Build history of the part. All positions in model axes, mm. Face numbers are marked on the shaded views. Give positions to 0.01 mm unless a question says otherwise; leave off trailing zeros. Write each loop counter-clockwise with the first axis right and the second up, starting at its lowest first coordinate (ties: lowest second). Pieces come first, ordered by that corner, then holes.
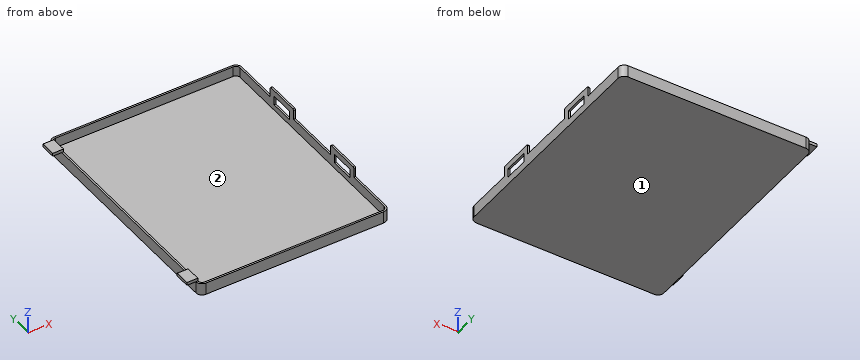
from build123d import *

# Parameters (mm, degrees)
BOSS_EXTRUDE1_DEPTH = 2
SHELL1_T            = -0.3
BOSS_EXTRUDE2_DEPTH = 0.3
SKETCH3_W           = 0.75
SKETCH3_H           = 4
CUT_EXTRUDE1_DEPTH  = 0.3
FILLET1_R           = 0.2
BOSS_EXTRUDE4_DEPTH = 0.5


with BuildPart() as part:
    # Sketch1 → Boss-Extrude1 (new body)
    with BuildSketch(Plane.XY):
        with BuildLine():
            Line((-14.75, 19.5), (14.75, 19.5))
            ThreePointArc((14.75, 19.5), (15.457106781, 19.207106781), (15.75, 18.5))
            Line((15.75, 18.5), (15.75, -18.5))
            ThreePointArc((15.75, -18.5), (15.457106781, -19.207106781), (14.75, -19.5))
            Line((14.75, -19.5), (-14.75, -19.5))
            ThreePointArc((-14.75, -19.5), (-15.457106781, -19.207106781), (-15.75, -18.5))
            Line((-15.75, -18.5), (-15.75, 18.5))
            ThreePointArc((-15.75, 18.5), (-15.457106781, 19.207106781), (-14.75, 19.5))
        make_face()
    extrude(amount=BOSS_EXTRUDE1_DEPTH)

    # Shell1
    shell1_openings = [part.faces().sort_by_distance(p)[0] for p in [
        (0, 0, 2),
    ]]
    offset(amount=SHELL1_T, openings=shell1_openings, kind=Kind.INTERSECTION)

    # Sketch2 → Boss-Extrude2 (add)
    with BuildSketch(Plane(origin=(15.75, 0, 0), x_dir=(0, 0, -1), z_dir=(1, 0, 0))):
        Polygon((-2, 10.75), (-3.75, 10.75), (-3.75, 4.75), (-2, 4.75), (-2, 5.75), (-2.75, 5.75), (-2.75, 9.75), (-2, 9.75), align=None)
    boss_extrude2 = extrude(amount=-BOSS_EXTRUDE2_DEPTH)

    # Mirror1: Boss-Extrude2 across plane
    add(boss_extrude2.mirror(Plane.ZX))

    # Sketch3 → Cut-Extrude1 (cut)
    with BuildSketch(Plane(origin=(15.75, 0, 0), x_dir=(0, 0, -1), z_dir=(1, 0, 0))):
        with Locations((-1.625, 7.75)):
            Rectangle(SKETCH3_W, SKETCH3_H)
        with Locations((-1.625, -7.75)):
            Rectangle(SKETCH3_W, SKETCH3_H)
    extrude(amount=-CUT_EXTRUDE1_DEPTH, mode=Mode.SUBTRACT)

    # Fillet1
    fillet1_edges = [part.edges().sort_by_distance(p)[0] for p in [
        (15.6, -10.75, 3.75),
        (15.6, 4.75, 3.75),
        (15.6, 10.75, 3.75),
        (15.6, -4.75, 3.75),
    ]]
    fillet(fillet1_edges, radius=FILLET1_R)

    # Sketch6 → Boss-Extrude4 (add)
    with BuildSketch(Plane.XY.offset(2)):
        Polygon((-17.25, -18.5), (-15.75, -18.5), (-15.45, -18.5), (-15.45, -16), (-15.75, -16), (-17.25, -16), align=None)
        Polygon((-17.25, 16), (-15.75, 16), (-15.45, 16), (-15.45, 18.5), (-15.75, 18.5), (-17.25, 18.5), align=None)
    extrude(amount=BOSS_EXTRUDE4_DEPTH)


solid = part.part
(1) Saw through at A-A, the plane y = -7.5. List the corners of the cut face in (x, z).
(2) Saw through at B-B, the plane y = 0.5. List the corners of the cut face in (x, z), plus the area to 3 significant figures.
(3) Mould opens along Y. For the marked faces 1 and 2 say: +Y half, -Y half, draft (parallel to the pull), parting line (faces both ways), or undercut.
(4) Saw through at C-C, the plane x = 1.5. List the corners of the cut face in (y, z), plus the area to 3 significant figures.
(5) Saw through at D-D, the plane y = -16.5. List the corners of the cut face in (x, z).
(6) Drop flat-ended pins along their axis: pin 1 (9.5 mm diameter, centred on x = 1, y = 16.5, fed in from +Z); pin 2 (1 mm diameter, centred on y = 0, z = 1.5, fed in from -X); pin 3 (9.5 mm diameter, centred on x = 3.5, y = -13, fed in from +Z). Give the stop position or say it passes through.
(7) Probe line 1 (X direction, y = -11, z = 1.7); line 2 (Y direction, x = -12, z = 0.35); line 3 (Z direction, x = 10, y = -13.5). List the from-to ranges inside material, lowest first.
Computed values:
1. outline: (-15.75, 0) - (15.75, 0) - (15.75, 1.25) - (15.45, 1.25) - (15.45, 0.3) - (-15.45, 0.3) - (-15.45, 2) - (-15.75, 2) - close; (15.45, 2.75) - (15.75, 2.75) - (15.75, 3.75) - (15.45, 3.75) - close
2. outline: (-15.75, 0) - (15.75, 0) - (15.75, 2) - (15.45, 2) - (15.45, 0.3) - (-15.45, 0.3) - (-15.45, 2) - (-15.75, 2) - close
2. area: 10.5 mm2
3. face 1: draft
3. face 2: undercut
4. outline: (-19.5, 0) - (19.5, 0) - (19.5, 2) - (19.2, 2) - (19.2, 0.3) - (-19.2, 0.3) - (-19.2, 2) - (-19.5, 2) - close
4. area: 12.7 mm2
5. outline: (-17.25, 2) - (-15.75, 2) - (-15.75, 0) - (15.75, 0) - (15.75, 2) - (15.45, 2) - (15.45, 0.3) - (-15.45, 0.3) - (-15.45, 2.5) - (-17.25, 2.5) - close
6. pin 1: stops at z = 2
6. pin 2: stops at x = -15.75
6. pin 3: stops at z = 0.3
7. line 1: x = -15.75 to -15.45, 15.45 to 15.75
7. line 2: y = -19.5 to -19.2, 19.2 to 19.5
7. line 3: z = 0 to 0.3
